Input: part model. Units: mm. Frame: model coordinates. Round coordinates to 2 decimals unless told otherwise and drop trailing zeros. Loops run counter-clockwise (first coordinate to the right, second up) from the corner with the lowest first, then second, coordinate; pieces in that order, holes last.
(1) Draft query along Z for faces 1 (the face through (30, 10, -90)), 2 (the face through (30, 10, 0)), 3 (the face through (56.735, 9.86, -87.194)), 4 (the face through (56.99, 9.86, -21.11)). Return one class per face: released by +Z, released by -Z, zero draft, split by the parting line, or undercut.
(2) Cut plane A-A, the plane x = 58. Output: boundary loops of the cut face in (y, z), and give its area (3 significant figures).
(3) Cut plane B-B, the plane z = -88. Output: boundary loops of the cut face in (x, y).
(4) Line query: line 1 (X direction, y = 8, z = -88); line 2 (Z direction, x = 58, y = 8.5). Output: solid intervals per line, ascending.
Autodesk Inventor part; units mm, degrees
ref_plane "YZ Plane" through (0, 0, 0) normal (1, 0, 0) x (0, 1, 0)
ref_plane "XZ Plane" through (0, 0, 0) normal (0, 1, 0) x (-1, 0, 0)
ref_plane "XY Plane" through (0, 0, 0) normal (0, 0, 1) x (1, 0, 0)
sketch "Skizze1" plane through (0, 0, 0) normal (0, 1, 0) x (-1, 0, 0)
  line L0 (0, 0) -> (-60, 0)
  line L1 (-60, 0) -> (-60, -90)
  line L2 (-60, -90) -> (0, -90)
  line L3 (0, -90) -> (0, 0)
  dimension "d0" = 60
  dimension "d1" = 90
extrude "Extrusion1" add sketch "Skizze1" along normal blind 20
sketch "Skizze2" plane through (0, 20, 0) normal (0, 1, 0) x (1, 0, 0)
  line L0 (60, 0) -> (60, 90)
  line L1 (60, 90) -> (0, 90)
  line L2 (0, 90) -> (0, 0)
  line L3 (0, 0) -> (60, 0)
  point P0 (58, 88)
  point P1 (2, 88)
  point P2 (2, 20)
  point P3 (58, 20)
  dimension "d4" = 2
  dimension "d5" = 2
  dimension "d6" = 2
  dimension "d7" = 2
  dimension "d8" = 2
  dimension "d9" = 2
  dimension "d10" = 20
  dimension "d11" = 20
hole "Bohrung1" at (58, 20, -88) at (58, 20, -20) at (2, 20, -88) at (2, 20, -20) direction (0, -1, 0) diameter 3 end through all
properties part number "Raspberry_Dummy"
Reported:
1. face 1: released by -Z
1. face 2: released by +Z
1. face 3: undercut
1. face 4: undercut
2. outline: (0, -90) - (20, -90) - (20, -89.5) - (0, -89.5) - close; (0, -86.5) - (20, -86.5) - (20, -21.5) - (0, -21.5) - close; (0, -18.5) - (20, -18.5) - (20, 0) - (0, 0) - close
2. area: 1,680 mm2
3. outline: (0, 0) - (0.5, 0) - (0.5, 20) - (0, 20) - close; (3.5, 0) - (56.5, 0) - (56.5, 20) - (3.5, 20) - close; (59.5, 0) - (60, 0) - (60, 20) - (59.5, 20) - close
4. line 1: x = 0 to 0.5, 3.5 to 56.5, 59.5 to 60
4. line 2: z = -90 to -89.5, -86.5 to -21.5, -18.5 to 0
